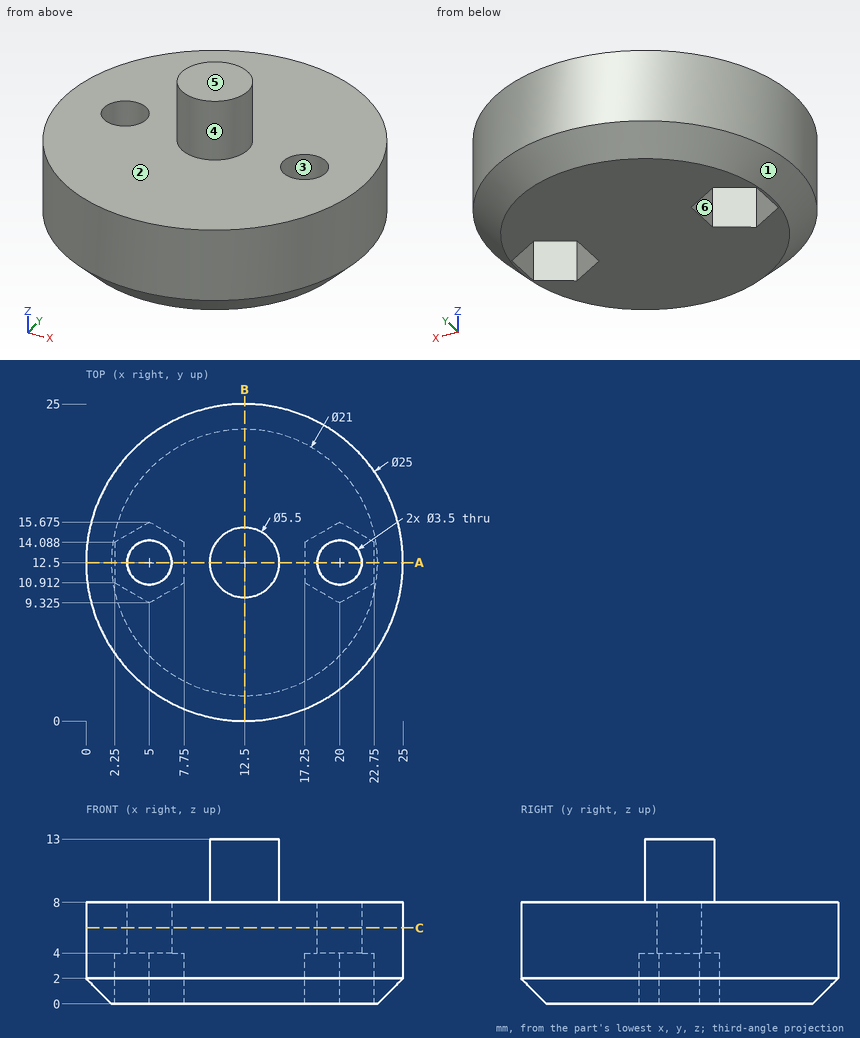
Here's the drawing with two shaded views (mm, measured from the low corner). I have some questions. A direction names the side the tool comes from. Round coordinates to 2 decimals unless told otherwise and drop trailing zeros. Loops run counter-clockwise (first coordinate to the right, second up) from the corner with the lowest first, then second, coordinate; pieces in that order, holes last. Notation, with made-up numbers: M 31.25,-31 L 62.25,-31 A22 ccw 62.25,-8 Z; hole C -28,66.5 d10. An arc over 180 degrees is marked long. Answer as a JSON object with one key per item and string values. Group by question number.
Q1. Imagine slicing it at B-B, the plane x = 12.5. Please give me the cut outline in (y, z).
Q2. Imagine slicing it at C-C, the plane z = 6. Please give me the cut outline in (x, y).
Q3. Imagine slicing it at A-A, the plane y = 12.5. Please give me the cut outline in (x, z).
Q4. We'd pull the mould along Y, two halves only. Please class the marked faces 1, 2 and 3: +Y half, -Y half, draft (parallel to the pull), parting line (faces both ways), or undercut.
Q5. Please list where these lines run through material, in increasing order: L1, parallel to Z at x = 3.75, y = 14.5; L2, parallel to Y at x = 5, z = 6.5; L3, parallel to Z at x = 11.5, y = 8.75.
Q6. On a 3-axis mill with a long thin cutter (end or side, diameter ignored), from which of +Z, -Z, +X, -X, +Y, -Y can I reach the whole of each face in a straight line? I mean the marked faces 4, 5 and 6. Say none if no direction works.
Q7. Will these pins go through, and if not, where does the flat tip stop? pin 1 (1.5 mm diameter, centred on x = 18.5, z = 6, fed in from +Y) (1 decimal); pin 2 (4.5 mm diameter, centred on x = 5, y = 12.5, fed in from +Z); pin 3 (3 mm diameter, centred on x = 20, y = 12.5, fed in from -Z); pin 4 (1 mm diameter, centred on x = 17.5, z = 5, fed in from -Y).
Findings:
{
 "1": {"outline": "M 0,2 L 2,0 L 23,0 L 25,2 L 25,8 L 15.25,8 L 15.25,13 L 9.75,13 L 9.75,8 L 0,8 Z"},
 "2": {"outline": "C 12.5,12.5 d25; hole C 5,12.5 d3.5; hole C 20,12.5 d3.5"},
 "3": {"outline": "M 0,2 L 2,0 L 2.25,0 L 2.25,4 L 3.25,4 L 3.25,8 L 0,8 Z; M 6.75,4 L 7.75,4 L 7.75,0 L 17.25,0 L 17.25,4 L 18.25,4 L 18.25,8 L 15.25,8 L 15.25,13 L 9.75,13 L 9.75,8 L 6.75,8 Z; M 21.75,4 L 22.75,4 L 22.75,0 L 23,0 L 25,2 L 25,8 L 21.75,8 Z"},
 "4": {"face 1": "parting line", "face 2": "draft", "face 3": "undercut"},
 "5": {"L1": "z = 4 to 8", "L2": "y = 2.5 to 10.75, 14.25 to 22.5", "L3": "z = 0 to 8"},
 "6": {"face 4": "+Z", "face 5": "+Z, +X, -X, +Y, -Y", "face 6": "-Z"},
 "7": {"pin 1": "stops at y = 23.8", "pin 2": "stops at z = 8", "pin 3": "passes through", "pin 4": "stops at y = 0.84"}
}
